For this review, use the dimensioned drawing (mm, ordinates from the lowest corner) and the shaded views. A direction names the side the tool comes from. Give positions to 0.01 mm unless a question says otherwise; leave off trailing zeros. Write each loop counter-clockwise with the first axis right and the second up, starting at its lowest first coordinate (ties: lowest second). Pieces come first, ordered by that corner, then holes. Notation, with made-up numbers: M 50.25,54 L 85.25,54 A36 cw 85.25,88 Z; hole C 53,44 d1. An arc over 180 degrees is marked long. One line per item, written item: value. Start each with the question number.
Item 1: Consider section C-C, the plane x = 16.51. Write out the cut boundary in (y, z), and give its area (3 significant figures).
Item 2: Consider section D-D, the plane x = 2. Write out the cut boundary in (y, z), and give its area (3 significant figures).
Item 3: Clearance check with flat-ended pins moving along their axes: pin 1 Ø7.5 at (y, z) = (12.7, 12.7) entering from -X; pin 2 Ø1 at (x, z) = (28.5, 20.5) entering from -Y; pin 3 Ø8 at (x, z) = (15, 18.5) entering from -Y; pin 4 Ø2 at (x, y) = (12, 62.5) entering from -Z. State where each tip first meets the part, or that it passes through.
Item 4: Consider section A-A, the plane y = 12.7. Write out the cut boundary in (x, z), and give its area (3 significant figures).
Item 5: Tool access review of the marked faces 1, 2 and 3: name each direction out of +Z, -Z, +X, -X, +Y, -Y from which nothing blocks a thin tool from reaching the whole face with its end or side.
Item 6: Mouldability with a two-part tool opening along Z and no side actions: class the marked faces 4, 5 and 6 as released by +Z, released by -Z, zero draft, split by the parting line, or undercut.
Item 7: To check wall thickness, follow probe 1 along Y at (x, z) = (28, 12.7); probe 2 along X at (y, z) = (25.5, 1); probe 3 along Z at (x, y) = (31, 12.7). State the ranges of each line that lie inside material, in increasing order.
Item 8: Consider section B-B, the plane z = 12.7. Write out the cut boundary in (x, y), and give its area (3 significant figures).
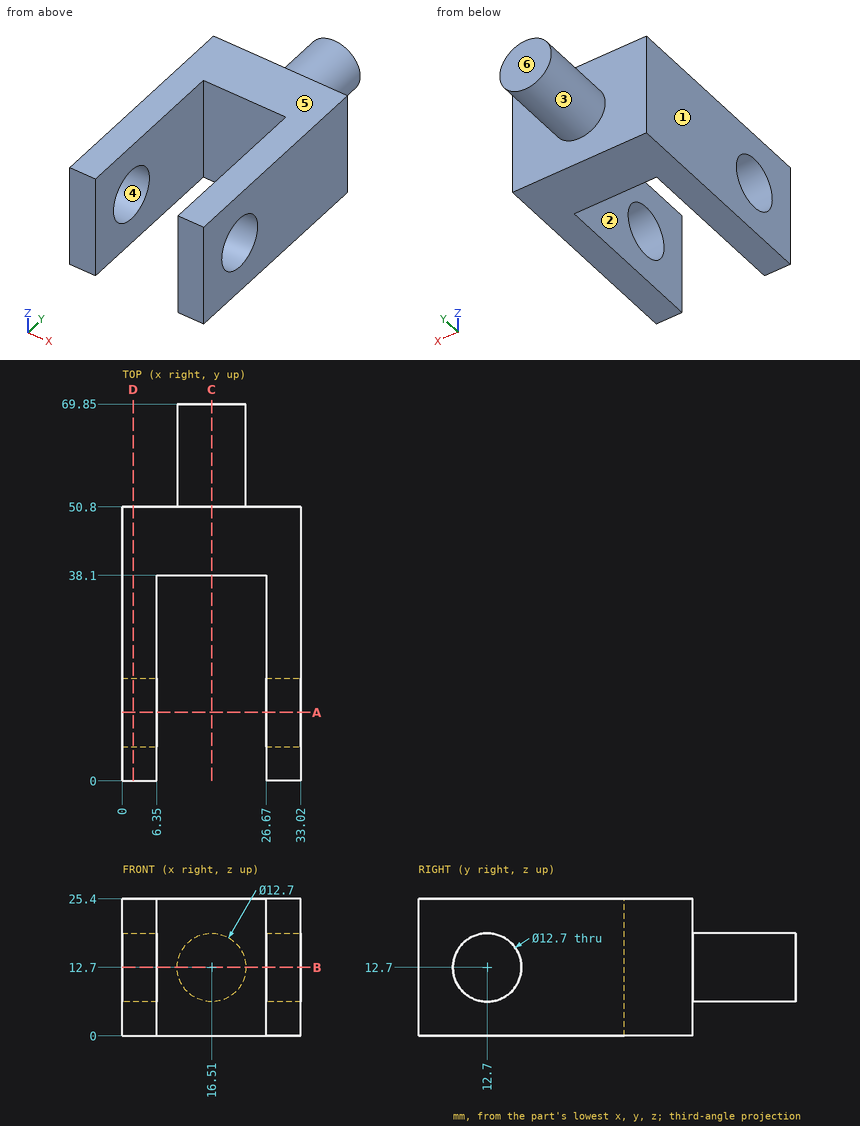
Model answer:
1. outline: M 38.1,0 L 50.8,0 L 50.8,6.35 L 69.85,6.35 L 69.85,19.05 L 50.8,19.05 L 50.8,25.4 L 38.1,25.4 Z
1. area: 565 mm2
2. outline: M 0,0 L 50.8,0 L 50.8,25.4 L 0,25.4 Z; hole C 12.7,12.7 d12.7
2. area: 1,160 mm2
3. pin 1: passes through
3. pin 2: stops at y = 0
3. pin 3: stops at y = 38.1
3. pin 4: stops at z = 7.41
4. outline: M 0,0 L 6.35,0 L 6.35,6.35 L 0,6.35 Z; M 0,19.05 L 6.35,19.05 L 6.35,25.4 L 0,25.4 Z; M 26.67,0 L 33.02,0 L 33.02,6.35 L 26.67,6.35 Z; M 26.67,19.05 L 33.02,19.05 L 33.02,25.4 L 26.67,25.4 Z
4. area: 161 mm2
5. face 1: +Z, -Z, -X, +Y, -Y
5. face 2: +Z, -Z, -Y
5. face 3: +Y
6. face 4: undercut
6. face 5: released by +Z
6. face 6: zero draft
7. probe 1: y = 0 to 6.35, 19.05 to 50.8
7. probe 2: x = 0 to 6.35, 26.67 to 33.02
7. probe 3: z = 0 to 6.35, 19.05 to 25.4
8. outline: M 0,0 L 6.35,0 L 6.35,6.35 L 0,6.35 Z; M 0,19.05 L 6.35,19.05 L 6.35,38.1 L 26.67,38.1 L 26.67,19.05 L 33.02,19.05 L 33.02,50.8 L 22.86,50.8 L 22.86,69.85 L 10.16,69.85 L 10.16,50.8 L 0,50.8 Z; M 26.67,0 L 33.02,0 L 33.02,6.35 L 26.67,6.35 Z
8. area: 984 mm2
